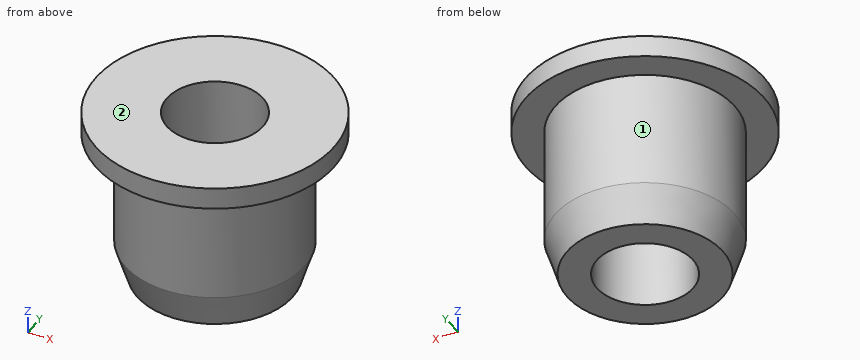
from build123d import *


# Not quite as in the source:
# - a feature names something its author has since deleted; it is built from what else it names


with BuildPart() as f1:
    # F0 (on Front) → F1 (revolve)
    with BuildSketch(Plane.XZ):
        Polygon((-13.335, 48.5521), (-32.97555, 48.5521), (-32.97555, 42.5196), (-24.8666, 42.5196), (-24.8666, 10.1854), (-21.5773, 0), (-13.335, 0), align=None)
    revolve(axis=Axis((0, 0, 24.27605), (0, 0, 1)))


solid = f1.part
Can you work these out from the model? Positions are in its coordinate system, mm. Face numbers are marked on the shaded views. A direction names the side the tool comes from. Give positions to 0.01 mm unless a question says otherwise; leave off trailing zeros. Order: outer loops, then holes, each group sorted by start corner. A loop starts at its lowest first (then second) coordinate and runs counter-clockwise, first axis right, second up. Notation, with made-up numbers: M 48.25,74 L 59.25,74 A7 ccw 59.25,78 Z; hole C 14.25,18.5 d5. An arc over 180 degrees is marked long. Use one line per item in the form item = value. Start each with the question number.
Item 1: If we section it at A-A (y = 0): Write out the boundary of the cut face in (x, z) (3 decimals).
Item 2: For the marked faces 1 and 2, which set-ups out of +Z, -Z, +X, -X, +Y, -Y let a thin tool reach every point of the face, with its end or its side?
Item 3: If we section it at C-C (z = 11.5): Write out the boundary of the cut face in (x, y) (3 decimals), then the cut area to 3 significant figures.
Item 4: Will these pins go through, and if not, where does the flat tip stop? pin 1 Ø1 at (x, y) = (-21, -23.5) entering from -Z; pin 2 Ø10 at (x, y) = (-2.5, 4.5) entering from +Z; pin 3 Ø12 at (y, z) = (-4.5, 29) entering from +X; pin 4 Ø3 at (x, z) = (-13.5, 34.5) entering from -Y.
Item 5: If I drill on line 1 along Y through (x, z) = (0, 16.5) (3 decimals); line 2 along Z through (x, y) = (-30, -3), over which ranges is the centre line in solid material (lowest first)?
Item 6: If we section it at D-D (y = -27): Write out the boundary of the cut face in (x, z).
Outcome:
q1.outline = M -32.976,42.52 L -24.867,42.52 L -24.867,10.185 L -21.577,0 L -13.335,0 L -13.335,48.552 L -32.976,48.552 Z; M 13.335,0 L 21.577,0 L 24.867,10.185 L 24.867,42.52 L 32.976,42.52 L 32.976,48.552 L 13.335,48.552 Z
q2.face_1 = -Z
q2.face_2 = +Z, +X, -X, +Y, -Y
q3.outline = C 0,0 d49.733; hole C 0,0 d26.67
q3.area = 1,380 mm2
q4.pin_1 = 42.52
q4.pin_2 = through
q4.pin_3 = 24.87
q4.pin_4 = -21.78
q5.line_1 = -24.867 to -13.335, 13.335 to 24.867
q5.line_2 = 42.52 to 48.55
q6.outline = M -18.93,42.52 L 18.93,42.52 L 18.93,48.55 L -18.93,48.55 Z
